Study the drawing (mm; zero at the part's minimum x, y, z) and answer. A direction names the side the tool comes from. Coordinates: 2 decimals unless noted, no trailing zeros. Order: outer loops, then holes, each group sorted by start corner. A loop starts at its lowest first (then second) coordinate and runs counter-clockwise, first axis right, second up.
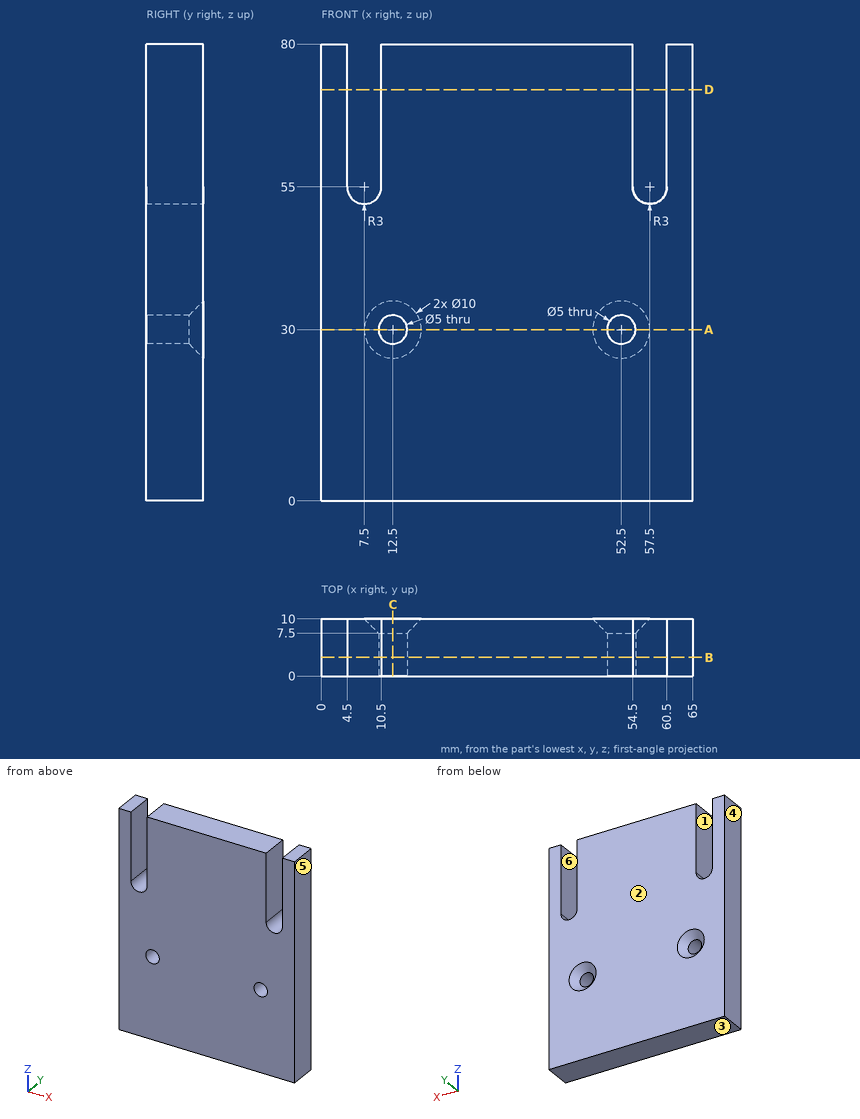
1) Straight lines are drawn through the part: line 1 (X direction, y = 5, z = 30); line 2 (X direction, y = 3, z = 63.5); line 3 (Z direction, x = 12.5, y = 2.5). For each, find the intervals that lie inside material, in ascending order.
A:
line 1: x = 0 to 10, 15 to 50, 55 to 65
line 2: x = 0 to 4.5, 10.5 to 54.5, 60.5 to 65
line 3: z = 0 to 27.5, 32.5 to 80
2) A cutting plane is placed at D-D, the plane z = 72. Determine the outline of the cut face in (x, y).
A:
outline: (0, 0) - (4.5, 0) - (4.5, 10) - (0, 10) - close; (10.5, 0) - (54.5, 0) - (54.5, 10) - (10.5, 10) - close; (60.5, 0) - (65, 0) - (65, 10) - (60.5, 10) - close
3) Which of the six approach directions +Z, -Z, +X, -X, +Y, -Y give full straight-line access (tool end or side, diameter ignored) to the marked faces 1 and 2?
A:
face 1: +Z, +Y, -Y
face 2: +Z, -Z, +X, -X, +Y
4) A cutting plane is placed at B-B, the plane y = 3.25. Determine the outline of the cut face in (x, z), and give its area (3 significant figures).
A:
outline: (0, 0) - (65, 0) - (65, 80) - (60.5, 80) - (60.5, 55) arc R3 cw to (54.5, 55) - (54.5, 80) - (10.5, 80) - (10.5, 55) arc R3 cw to (4.5, 55) - (4.5, 80) - (0, 80) - close; hole circle Ø5 at (12.5, 30); hole circle Ø5 at (52.5, 30)
area: 4,830 mm2
5) A cutting plane is placed at A-A, the plane z = 30. Determine the outline of the cut face in (x, y), and give its area (4 significant figures).
A:
outline: (0, 0) - (10, 0) - (10, 7.5) - (7.5, 10) - (0, 10) - close; (15, 0) - (50, 0) - (50, 7.5) - (47.5, 10) - (17.5, 10) - (15, 7.5) - close; (55, 0) - (65, 0) - (65, 10) - (57.5, 10) - (55, 7.5) - close
area: 537.5 mm2
6) A cutting plane is placed at C-C, the plane x = 12.5. Determine the outline of the cut face in (y, z), and give its area (3 significant figures).
A:
outline: (0, 0) - (10, 0) - (10, 25) - (7.5, 27.5) - (0, 27.5) - close; (0, 32.5) - (7.5, 32.5) - (10, 35) - (10, 80) - (0, 80) - close
area: 744 mm2
7) Determine the mould class of the marked faces 3, 4, 5 and 6 for opening direction X: pulls with the +X half, pulls with the -X half, needs draft (parallel to the pull), parting line crosses it, or undercut.
A:
face 3: needs draft
face 4: pulls with the -X half
face 5: pulls with the +X half
face 6: undercut
